Source: three-view drawing plus pictorial views. Frame: mm from the lowest corner of the part. Give positions to 0.01 mm unless a question says otherwise; leave off trailing zeros. Loops run counter-clockwise (first coordinate to the right, second up) from the corner with the lowest first, then second, coordinate; pieces in that order, holes last. Notation, with made-up numbers: (79.5, 81.25) - (87.5, 81.25) arc R26 cw to (87.5, 116.25) - close; hole circle Ø3 at (86, 72.5). An arc over 180 degrees is marked (long way). Answer in a Markdown table with one row per item.
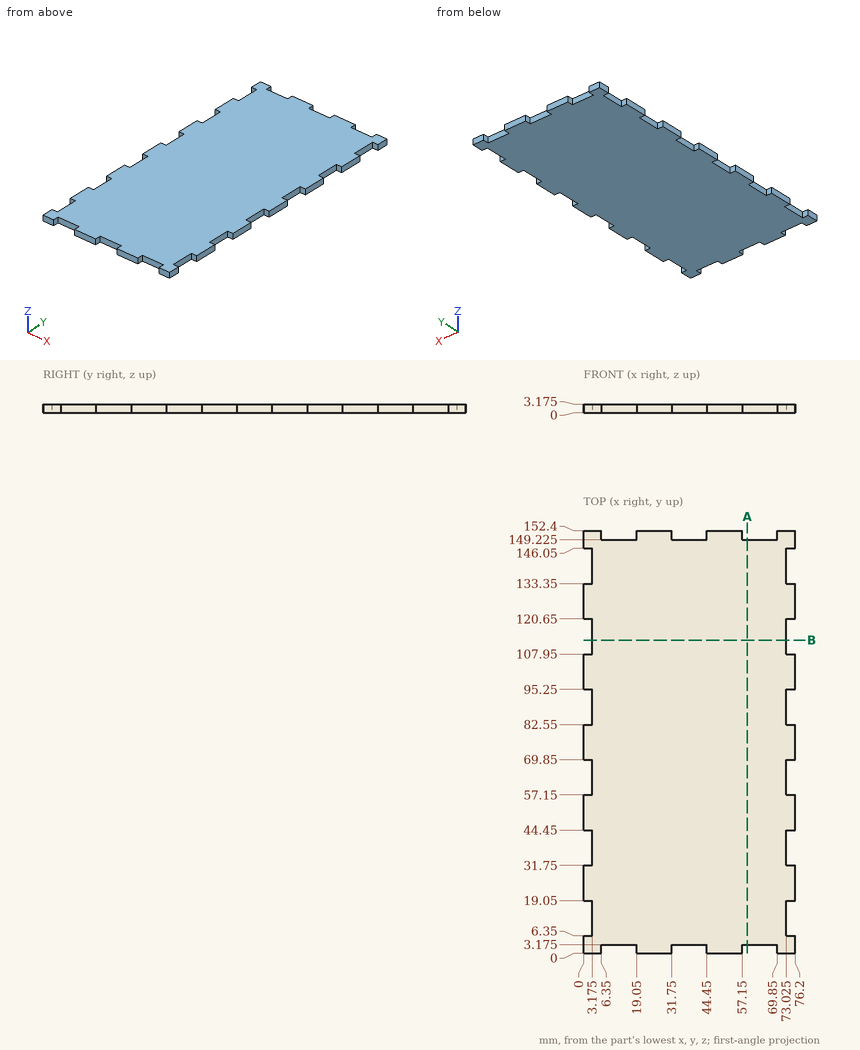
Q1. Material intervals for line 1 along Y through (x, z) = (67.5, 0.5) (3 decimals); line 2 along X through (y, z) = (85, 0.65) (3 decimals), sorted ascending.
Check values:
| item | result |
|---|---|
| line 1 | 3.175 to 149.225 |
| line 2 | 3.175 to 73.025 |
Q2. Cut plane A-A (x = 59). Output: boundary loops of the cut face in (y, z) (3 decimals), and give its area (3 significant figures).
Check values:
| item | result |
|---|---|
| outline | (3.175, 0) - (149.225, 0) - (149.225, 3.175) - (3.175, 3.175) - close |
| area | 464 mm² |
Q3. First-contact query: pin 1 (6 mm diameter, centred on x = 44, y = 35, fed in from -Z); pin 2 (1.6 mm diameter, centred on x = 36, z = 1.5, fed in from +Y) (3 decimals); pin 3 (1.6 mm diameter, centred on y = 89.5, z = 1.5, fed in from +X) (3 decimals). Flat tips, straight axial feed; report the tip coordinate or a pass-through.
Check values:
| item | result |
|---|---|
| pin 1 | z = 0 |
| pin 2 | y = 149.225 |
| pin 3 | x = 73.025 |
Q4. Cut plane B-B (y = 113). Output: boundary loops of the cut face in (x, z) (3 decimals), and give its area (3 significant figures).
Check values:
| item | result |
|---|---|
| outline | (3.175, 0) - (73.025, 0) - (73.025, 3.175) - (3.175, 3.175) - close |
| area | 222 mm² |
